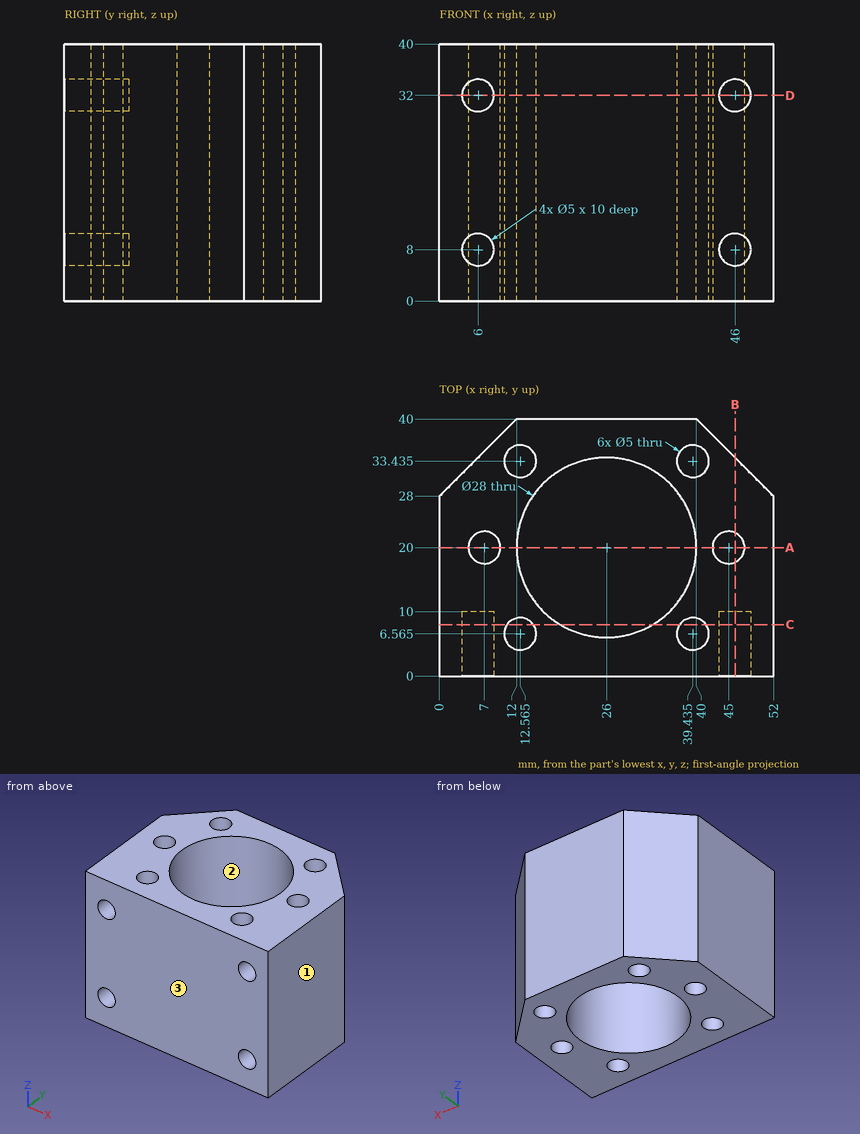
Check sheet for the drawn part. Datum: minimum x, y, z corner. Units: mm. Give positions to 0.01 mm unless a question says otherwise; leave off trailing zeros. Order: outer loops, then holes, each group sorted by start corner. A loop starts at its lowest first (then second) coordinate and runs counter-clockwise, first axis right, second up. Notation, with made-up numbers: (34.5, 50) - (44.5, 50) arc R21 cw to (44.5, 57) - close; hole circle Ø3 at (33.25, 42). An arc over 180 degrees is marked (long way). Write item = value, one per line. Start each with the question number.
1) Section check D-D (z = 32). Enter the section's corners in (x, y) (3 decimals), then the cut area to 3 significant figures.
2) Section check B-B (x = 46). Enter the section's corners in (y, z).
3) Draft check along X on the marked faces 1, 2 and 3. Enter one of: released by +X, released by -X, zero draft, split by the parting line, or undercut.
4) Section check A-A (y = 20). Enter the section's corners in (x, z).
5) Section check C-C (y = 8). Enter the section's corners in (x, z), then the cut area to 3 significant figures.
6) Gauge pin test, flat ends, axial feed: pin 1 Ø4 at (x, z) = (46, 32) entering from -Y; pin 2 Ø5.5 at (x, z) = (7, 8.5) entering from -Y; pin 3 Ø4 at (x, y) = (39.435, 33.435) entering from -Z. Record the tip position at first contact, or that the pin passes through.
7) Scan lines: L1, parallel to Z at x = 46, y = 5; L2, parallel to X at y = 22, z = 20; L3, parallel to Y at x = 38.5, z = 26. Record each from-to range of solid material in increasing order.
Geometry check:
q1.outline = (0, 0) - (3.5, 0) - (3.5, 10) - (8.5, 10) - (8.5, 0) - (43.5, 0) - (43.5, 10) - (48.5, 10) - (48.5, 0) - (52, 0) - (52, 28) - (40, 40) - (12, 40) - (0, 28) - close; hole circle Ø5 at (7, 20); hole circle Ø5 at (12.565, 6.565); hole circle Ø5 at (12.565, 33.435); hole circle Ø28 at (26, 20); hole circle Ø5 at (39.435, 6.565); hole circle Ø5 at (39.435, 33.435); hole circle Ø5 at (45, 20)
q1.area = 1,100 mm2
q2.outline = (0, 0) - (17.71, 0) - (17.71, 40) - (0, 40) - (0, 34.5) - (10, 34.5) - (10, 29.5) - (0, 29.5) - (0, 10.5) - (10, 10.5) - (10, 5.5) - (0, 5.5) - close; (22.29, 0) - (34, 0) - (34, 40) - (22.29, 40) - close
q3.face_1 = released by +X
q3.face_2 = undercut
q3.face_3 = zero draft
q4.outline = (0, 0) - (4.5, 0) - (4.5, 40) - (0, 40) - close; (9.5, 0) - (12, 0) - (12, 40) - (9.5, 40) - close; (40, 0) - (42.5, 0) - (42.5, 40) - (40, 40) - close; (47.5, 0) - (52, 0) - (52, 40) - (47.5, 40) - close
q5.outline = (0, 0) - (10.52, 0) - (10.52, 40) - (0, 40) - close; (14.61, 0) - (18.79, 0) - (18.79, 40) - (14.61, 40) - close; (33.21, 0) - (37.39, 0) - (37.39, 40) - (33.21, 40) - close; (41.48, 0) - (52, 0) - (52, 40) - (41.48, 40) - close; hole circle Ø5 at (6, 8); hole circle Ø5 at (6, 32); hole circle Ø5 at (46, 8); hole circle Ø5 at (46, 32)
q5.area = 1,100 mm2
q6.pin_1 = 10
q6.pin_2 = 0
q6.pin_3 = through
q7.L1 = 0 to 5.5, 10.5 to 29.5, 34.5 to 40
q7.L2 = 0 to 5.5, 8.5 to 12.14, 39.86 to 43.5, 46.5 to 52
q7.L3 = 0 to 4.25, 8.88 to 13.7, 26.3 to 31.12, 35.75 to 40
